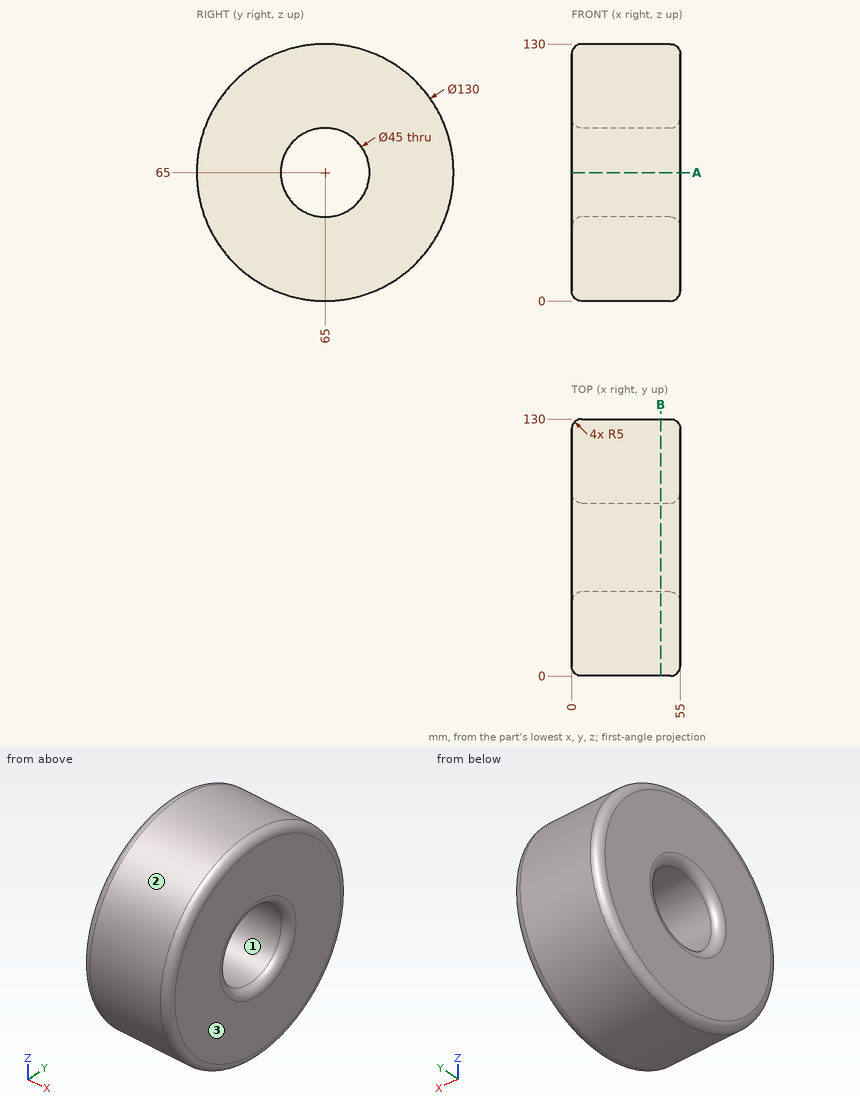
Study the drawing (mm; zero at the part's minimum x, y, z) and answer. Give positions to 0.01 mm unless a question says otherwise; leave off trailing zeros. Order: outer loops, then holes, each group sorted by start corner. A loop starts at its lowest first (then second) coordinate and runs counter-clockwise, first axis right, second up.
1. Section B-B, the plane x = 45 is taken. Determine the outline of the cut face in (y, z).
Result sheet:
outline: circle Ø130 at (65, 65); hole circle Ø45 at (65, 65)
2. Each of these flat-tipped pins is pushed along its axis until it touches: P1, Ø12, axis at x = 34.5, z = 79, coming from the -Y side; P2, Ø3, axis at x = 7.5, z = 39.5, coming from the +Y side; P3, Ø10, axis at x = 47.5, z = 102.5, coming from the -Y side. Where does it stop, or does it pass through?
Result sheet:
P1: stops at y = 0.49
P2: stops at y = 125.41
P3: stops at y = 8.71
3. Straight lines are drawn through the part: L1, parallel to Z at x = 15, y = 65; L2, parallel to X at y = 8.5, z = 86; L3, parallel to Y at x = 30, z = 51.5. For each, find the intervals that lie inside material, in ascending order.
Result sheet:
L1: z = 0 to 42.5, 87.5 to 130
L2: x = 0.01 to 54.99
L3: y = 1.42 to 47, 83 to 128.58
4. Section A-A, the plane z = 65 is taken. Determine the outline of the cut face in (x, y).
Result sheet:
outline: (0, 5) arc R5 ccw to (5, 0) - (50, 0) arc R5 ccw to (55, 5) - (55, 37.5) arc R5 ccw to (50, 42.5) - (5, 42.5) arc R5 ccw to (0, 37.5) - close; (0, 92.5) arc R5 ccw to (5, 87.5) - (50, 87.5) arc R5 ccw to (55, 92.5) - (55, 125) arc R5 ccw to (50, 130) - (5, 130) arc R5 ccw to (0, 125) - close
5. The mould has two halves that part along Z. Classify the marked faces 1, 2 and 3: released by +Z, released by -Z, zero draft, split by the parting line, or undercut.
Result sheet:
face 1: undercut
face 2: split by the parting line
face 3: zero draft
